For this review, take the finished solid that the model builds, in its own axes (mm). A direction names the side the tool comes from. Give positions to 0.01 mm unless a question says otherwise; leave off trailing zeros. Loops run counter-clockwise (first coordinate to the right, second up) from the corner with the lowest first, then second, coordinate; pieces in that order, holes last. Notation, with made-up numbers: M 65.25,12 L 113.25,12 A17 cw 113.25,28 Z; hole C 15.25,-23.75 d3. An arc over 180 degrees is marked long. Use CSV: the item, a comma, the result in double quotes. Start each with the question number.
1. Tool access review of faces 1 (the face through (2, 0, 6.5)), 2 (the face through (51, 5, -4.5)), 3 (the face through (50.6, -5.9, 2.1)): name each direction out of +Z, -Z, +X, -X, +Y, -Y from which nothing blocks a thin tool from reaching the whole face with its end or side.
2. Take a section at B-B, the plane y = -3. Write out the cut boundary in (x, z), and give its area (3 significant figures).
3. Take a section at A-A, the plane z = 5.25. Write out the cut boundary in (x, y), and give its area (3 significant figures).
4. Take a section at C-C, the plane y = 6. Write out the cut boundary in (x, z).
5. The part is to be moulded in two halves that separate along X. For faces 4 (the face through (13, 4.999, -5)), 5 (the face through (50.12, 6.32, 1.33)), say which applies: pulls with the +X half, pulls with the -X half, needs draft (parallel to the pull), parting line crosses it, or undercut.
6. To check wall thickness, follow line 1 (X direction, y = -1, z = 3.75); line 2 (Y direction, x = 52, z = -4.25); line 3 (Y direction, x = 13, z = -4.5). State the ranges of each line that lie inside material, in increasing order. Write a range as [from, to].
7. Take a section at D-D, the plane x = 28. Write out the cut boundary in (y, z).
8. Insertion check: P1, Ø8, axis at x = -2, y = 1.5, coming from the +Z side; P2, Ø4, axis at x = 42, y = -8.5, coming from the +Z side; P3, Ø4, axis at x = 0, y = 0, coming from the -Z side; P4, Ø6, axis at y = 12.5, z = 3.5, coming from the -X side. Each pin has a flat end and moves straight along its axis. Give the tip position at first contact, or say it passes through.
from build123d import *
from build123d.topology import SkipClean

# Parameters (mm, degrees)
BOSS_EXTRU_1_DEPTH      = 7
BOSS_EXTRU_1_DEPTH_BACK = 7
ESQUISSE1_R             = 1.55
ESQUISSE3_R             = 7.5
ESQUISSE3_R_2           = 4.5
ENL_V_MAT_EXTRU_1_DEPTH = 12
ENL_V_MAT_EXTRU_2_REACH = 61.679
ESQUISSE5_R             = 1.55
ENL_V_MAT_EXTRU_3_DEPTH = 14
ENL_V_MAT_EXTRU_4_DEPTH = 11.5
ENL_V_MAT_EXTRU_5_DEPTH = 10
ESQUISSE8_R             = 5
ESQUISSE8_R_2           = 1.55
BOSS_EXTRU_3_DEPTH      = 9.5
SKETCH1_R               = 1.55
CUT_EXTRUDE1_DEPTH      = 14


with BuildPart() as part:
    # Esquisse1 → Boss.-Extru.1 (new, two sides: drawn at the far end of the back side and taken through both)
    with BuildSketch(Plane.XY.offset(-BOSS_EXTRU_1_DEPTH_BACK)):
        with BuildLine():
            Line((-0.121307676, 4.998528228), (26.897812493, 4.998528228))
            ThreePointArc((26.897812493, 4.998528228), (43.36686221, 14.818498296), (56.034466428, 0.42429064))
            ThreePointArc((56.034466428, 0.42429064), (43.785088024, -14.746764493), (26.897812493, -4.998528228))
            Line((26.897812493, -4.998528228), (-0.121307676, -4.998528228))
            ThreePointArc((-0.121307676, -4.998528228), (-5, 0), (-0.121307676, 4.998528228))
        make_face()
        Circle(ESQUISSE1_R, mode=Mode.SUBTRACT)
    extrude(amount=BOSS_EXTRU_1_DEPTH + BOSS_EXTRU_1_DEPTH_BACK)

    # Esquisse3 → Enlèv. mat.-Extru.1 (cut)
    with BuildSketch(Plane.XY.offset(7)):
        with Locations((41.040468381, 0)):
            Circle(ESQUISSE3_R)
        with Locations((41.040468381, 0)):
            Circle(ESQUISSE3_R_2, mode=Mode.SUBTRACT)
    extrude(amount=-ENL_V_MAT_EXTRU_1_DEPTH, mode=Mode.SUBTRACT)

    # Enlèv. mat.-Extru.2: up to this face of the body (flat: up to its plane)
    enl_v_mat_extru_2_end = Plane(part.part.faces().sort_by_distance((32.334245268, 0, -7))[0])
    # Esquisse4 → Enlèv. mat.-Extru.2 (cut, up to the picked face)
    with BuildSketch(Plane.XY.offset(7), mode=Mode.PRIVATE) as enl_v_mat_extru_2_sk1:
        with BuildLine():
            Line((26.897812493, 4.998528228), (33.969140437, 2.499264114))
            ThreePointArc((33.969140437, 2.499264114), (37.833778623, 6.779907138), (43.594458809, 7.051746797))
            Line((43.594458809, 7.051746797), (43.594458809, 14.780971987))
            ThreePointArc((43.594458809, 14.780971987), (33.45770218, 12.942243111), (26.897812493, 4.998528228))
        make_face()
    enl_v_mat_extru_2_tool1 = split(extrude(enl_v_mat_extru_2_sk1.sketch, amount=-ENL_V_MAT_EXTRU_2_REACH, mode=Mode.PRIVATE), bisect_by=enl_v_mat_extru_2_end, keep=Keep.BOTH, mode=Mode.PRIVATE)
    add(enl_v_mat_extru_2_tool1.solids().sort_by(Axis((35.915209, 9.281231, 7), (0, 0, -1)))[0], mode=Mode.SUBTRACT)

    # Esquisse5 → Enlèv. mat.-Extru.3 (cut)
    with BuildSketch(Plane.XY.offset(7)):
        with Locations((41.040468381, 0)):
            Circle(ESQUISSE5_R)
    extrude(amount=-ENL_V_MAT_EXTRU_3_DEPTH, mode=Mode.SUBTRACT)

    # Esquisse6 → Enlèv. mat.-Extru.4 (cut)
    with BuildSketch(Plane(origin=(0, 0, 7), x_dir=(-1, 0, 0), z_dir=(0, 0, -1))):
        with BuildLine():
            Line((-47.967646393, 2.874752996), (-52.337500651, 9.867981652))
            ThreePointArc((-52.337500651, 9.867981652), (-53.013141031, 9.036321686), (-53.627686287, 8.158550445))
            Line((-53.627686287, 8.158550445), (-48.540448501, 0.017268159))
            ThreePointArc((-48.540448501, 0.017268159), (-48.394176822, 1.474100456), (-47.967646393, 2.874752996))
        make_face()
    extrude(amount=ENL_V_MAT_EXTRU_4_DEPTH, mode=Mode.SUBTRACT)

    # Esquisse7 → Enlèv. mat.-Extru.5 (cut)
    with BuildSketch(Plane.XY.offset(7)):
        with BuildLine():
            Line((47.423042191, -3.938623052), (53.805616002, -7.877246105))
            ThreePointArc((53.805616002, -7.877246105), (39.444806634, -14.914887314), (26.897812493, -4.998528228))
            Line((26.897812493, -4.998528228), (-0.121307676, -4.998528228))
            ThreePointArc((-0.121307676, -4.998528228), (-5.242615351, 0), (-0.121307676, 4.998528228))
            Line((-0.121307676, 4.998528228), (26.897812493, 4.998528228))
            Line((26.897812493, 4.998528228), (33.969140437, 2.499264114))
            ThreePointArc((33.969140437, 2.499264114), (37.803155706, -6.76533862), (47.423042191, -3.938623052))
        make_face()
    extrude(amount=-ENL_V_MAT_EXTRU_5_DEPTH, mode=Mode.SUBTRACT)

    # Esquisse8 → Boss.-Extru.3 (add)
    with SkipClean():  # the faces are left unmerged after this step: merging them gives an invalid solid
        with BuildSketch(Plane.XY.offset(-3)):
            Circle(ESQUISSE8_R)
            Circle(ESQUISSE8_R_2, mode=Mode.SUBTRACT)
        extrude(amount=BOSS_EXTRU_3_DEPTH)

    # Sketch1 → Cut-Extrude1 (cut)
    with SkipClean():  # the faces are left unmerged after this step: merging them gives an invalid solid
        with BuildSketch(Plane.XY.offset(7)):
            with Locations((52.040468381, -3)):
                Circle(SKETCH1_R)
        extrude(amount=-CUT_EXTRUDE1_DEPTH, mode=Mode.SUBTRACT)


solid = part.part
Result set:
1,face 1,"+Z, -X, +Y, -Y"
1,face 2,"+Z"
1,face 3,"+Z, -Y"
2,outline,"M -4,-7 L 50.49,-7 L 50.49,7 L 47.91,7 L 47.91,-5 L 44.39,-5 L 44.39,7 L 37.69,7 L 37.69,-5 L 34.17,-5 L 34.17,-3 L 4,-3 L 4,6.5 L -4,6.5 Z; M 53.59,-7 L 55.74,-7 L 55.74,7 L 53.59,7 Z"
2,area,"403 mm2"
3,outline,"C 0,0 d10; C 41.04,0 d9; M 43.59,7.05 A7.5 cw 47.97,2.87 L 52.34,9.87 A15 ccw 43.59,14.78 Z; M 47.42,-3.94 L 53.81,-7.88 A15 ccw 53.63,8.16 L 48.54,0.02 A7.5 cw Z; hole C 0,0 d3.1; hole C 41.04,0 d3.1; hole C 52.04,-3 d3.1"
3,area,"262 mm2"
4,outline,"M 36.54,-7 L 54.79,-7 L 54.79,7 L 52.28,7 L 52.28,-4.5 L 49.92,-4.5 L 49.92,7 L 45.54,7 L 45.54,-5 L 36.54,-5 Z"
5,face 4,"needs draft"
5,face 5,"undercut"
6,line 1,"[-4.9, -1.18], [1.18, 4.9], [36.65, 39.86], [42.22, 45.43], [48.47, 56.01]"
6,line 2,"[-10.24, -4.55], [-1.45, 5.55], [9.33, 10.24]"
6,line 3,"[-5, 5]"
7,outline,"M -7.41,-7 L 4.61,-7 L 4.61,-3 L -7.41,-3 Z"
8,P1,"z = 6.5"
8,P2,"z = -3"
8,P3,"z = -7"
8,P4,"x = 43.59"
